For this review, take the finished solid that the model builds, in its own axes (mm). A direction names the side the tool comes from. Round coordinates to 2 decimals unless told otherwise and drop trailing zeros. Order: outer loops, then holes, each group sorted by start corner. A loop starts at its lowest first (then second) coordinate and runs counter-clockwise, first axis right, second up. Notation, with made-up numbers: (52, 44.5) - (64, 44.5) arc R12 cw to (64, 48.5) - close; hole circle Ø1 at (48.5, 10.5). An arc over 180 degrees is marked (long way). One line per item, written item: value.
```python
from build123d import *

# Parameters (mm, degrees)
SKETCH_R     = 5
PAD_DEPTH    = 8
SKETCH001_R  = 18
POCKET_DEPTH = 8.001


with BuildPart() as part:
    # Sketch → Pad (new body)
    with BuildSketch(Plane.XZ):
        Polygon((0, 0), (50, 0), (50, -50), (100, -50), (100, 0), (150, 0), (150, 120), (100, 170), (50, 170), (0, 120), align=None)
        with Locations((75, -25)):
            Circle(SKETCH_R, mode=Mode.SUBTRACT)
    extrude(amount=PAD_DEPTH)

    # Sketch001 → Pocket (cut, through all)
    with BuildSketch(Plane.XZ):
        with Locations((75, 110)):
            Circle(SKETCH001_R)
    extrude(amount=POCKET_DEPTH, mode=Mode.SUBTRACT)


solid = part.part
```
Item 1: Take a section at A-A (z = -25). Write out the cut boundary in (x, y), plus the area to 3 significant figures.
Returned:
outline: (50, -8) - (70, -8) - (70, 0) - (50, 0) - close; (80, -8) - (100, -8) - (100, 0) - (80, 0) - close
area: 320 mm^2
Item 2: Machinability: for faces 5 (the flat face through (74, -8, 62)), 6 (the flat face through (125, -4, 0)), 7 (the flat face through (25, -4, 0)), which of the approach directions +Z, -Z, +X, -X, +Y, -Y give a long, thin tool a straight path to every point of the face, cutting with its end or side? Answer none if there is none.
Returned:
face 5: +Z, -Z, +X, -X, -Y
face 6: -Z, +X, +Y, -Y
face 7: -Z, -X, +Y, -Y
Item 3: Take a section at C-C (y = -4.5). Write out the cut boundary in (x, z).
Returned:
outline: (0, 0) - (50, 0) - (50, -50) - (100, -50) - (100, 0) - (150, 0) - (150, 120) - (100, 170) - (50, 170) - (0, 120) - close; hole circle Ø36 at (75, 110); hole circle Ø10 at (75, -25)
Item 4: For P1, Ø4, axis at y = -4, z = -15, coming from the +X side; P2, Ø4, axis at y = -5.5, z = -15, coming from the -X side, all flat-tipped, find the tip position at first contact; note any pin that passes through.
Returned:
P1: x = 100
P2: x = 50
Item 5: The part is to be moulded in two halves that separate along X. For faces 1 (the cylindrical face through (79.619, -3.944, -26.915)), 2 (the flat face through (50, -4, -25)), 3 (the cylindrical face through (61.733, -3.944, 122.165)), 4 (the flat face through (75, -4, 170)), say which applies: +X half, -X half, draft (parallel to the pull), parting line (faces both ways), or undercut.
Returned:
face 1: undercut
face 2: -X half
face 3: undercut
face 4: draft
Item 6: Take a section at D-D (z = 110). Write out the cut boundary in (x, y), plus the area to 3 significant figures.
Returned:
outline: (0, -8) - (57, -8) - (57, 0) - (0, 0) - close; (93, -8) - (150, -8) - (150, 0) - (93, 0) - close
area: 912 mm^2
Item 7: Take a section at B-B (x = 75). Write out the cut boundary in (y, z).
Returned:
outline: (-8, -50) - (0, -50) - (0, -30) - (-8, -30) - close; (-8, -20) - (0, -20) - (0, 92) - (-8, 92) - close; (-8, 128) - (0, 128) - (0, 170) - (-8, 170) - close
Item 8: Wall thickness on line 1 (Z direction, x = 75, y = -3.25); line 2 (Z direction, x = 78, y = -1.5); line 3 (X direction, y = -1, z = -34.5): over which ranges is each line inside the solid? List them lowest first.
Returned:
line 1: -50 to -30, -20 to 92, 128 to 170
line 2: -50 to -29, -21 to 92.25, 127.75 to 170
line 3: 50 to 100
